```python
from build123d import *

# Parameters (mm, degrees)
F1_DEPTH = 81.5
F2_W     = 1.85
F2_H     = 25.8
F2_H_2   = 4.1
F3_DEPTH = 1.95
F2_W_2   = 7
F4_DEPTH = 8
F5_START = 5
F5_DEPTH = 3


with BuildPart() as f1:
    # F0 (on Top) → F1 (new body)
    with BuildSketch(Plane.XY):
        Polygon((0, -55.5), (0, 0), (10, 0), (10, 9.5), (-5, 9.5), (-5, -50.5), (-80, -50.5), (-80, 9.5), (-95, 9.5), (-95, 0), (-85, 0), (-85, -55.5), align=None)
    extrude(amount=F1_DEPTH)

    # F2 (on face) → F3 (join)
    with BuildSketch(Plane(origin=(0, -50.5, 0), x_dir=(-1, 0, 0), z_dir=(0, 1, 0))):
        Polygon((42.5, 47.4), (42.5, 51.5), (40.65, 51.5), (40.65, 17.5), (42.5, 17.5), (42.5, 21.6), align=None)
        with Locations((43.425, 34.5)):
            Rectangle(F2_W, F2_H)
        with Locations((43.425, 49.45)):
            Rectangle(F2_W, F2_H_2)
        with Locations((43.425, 19.55)):
            Rectangle(F2_W, F2_H_2)
    extrude(amount=F3_DEPTH)

    # F2 (on face) → F4 (join)
    with BuildSketch(Plane(origin=(0, -50.5, 0), x_dir=(-1, 0, 0), z_dir=(0, 1, 0))):
        with Locations((61, 34.5)):
            Rectangle(F2_W_2, F2_H)
        with Locations((24, 34.5)):
            Rectangle(F2_W_2, F2_H)
    extrude(amount=F4_DEPTH)

    # F2 (on face) → F5 (join)
    with BuildSketch(Plane(origin=(0, -50.5, 0), x_dir=(-1, 0, 0), z_dir=(0, 1, 0)).offset(F5_START)):
        Polygon((29.95, 24.05), (29.95, 44.95), (27.5, 47.4), (27.5, 21.6), align=None)
        Polygon((57.5, 21.6), (57.5, 47.4), (55.05, 44.95), (55.05, 24.05), align=None)
    extrude(amount=F5_DEPTH)


solid = f1.part
```
Here's how the part is built. I have some questions about the finished solid (model axes, mm). A direction names the side the tool comes from. Give positions to 0.01 mm unless a question says otherwise; leave off trailing zeros. Order: outer loops, then holes, each group sorted by start corner. A loop starts at its lowest first (then second) coordinate and runs counter-clockwise, first axis right, second up. Notation, with made-up numbers: M 32.25,42 L 68.25,42 A21 ccw 68.25,79 Z; hole C -36,20 d5. An arc over 180 degrees is marked long. Use a Markdown table: item, result. Add a question column.
1. Suppose I cut it at D-D (z = 77). List the corners of the cut face in (x, y) for me, and give its area (4 significant figures).
2. If we mould it in two halves opening along Y, with no side actions, what happens to faces 1 (the flat face through (-64.5, -47, 34)), 2 (the flat face through (-57.5, -48, 34)), 3 (the flat face through (-42, -48.55, 35))? For each: +Y half, -Y half, draft (parallel to the pull), parting line (faces both ways), or undercut.
3. Suppose I cut it at B-B (x = -23). List the corners of the cut face in (y, z) for me.
4. For pin 1 Ø4 at (y, z) = (-45, 33.5) entering from +X; pin 2 Ø1 at (y, z) = (-33, 22) entering from -X; pin 3 Ø4 at (x, z) = (-41.5, 42) entering from +Y; pin 4 Ø6 at (x, y) = (-52.5, -38) entering from +Z, each with a flat end and sliding along its axis, tell me the tip position at first contact or that it passes through.
5. I need wall thicknesses on probe 1 along X at (y, z) = (-21, 28.5); probe 2 along X at (y, z) = (1.5, 41.5); probe 3 along Y at (x, z) = (2.5, 77.5). Which ranges of each line are inside material? Lowest first, please. Write a range as from..to.
6. Suppose I cut it at A-A (y = -9). List the corners of the cut face in (x, z) for me, and give its area (3 significant figures).
7. Suppose I cut it at C-C (z = 39). List the corners of the cut face in (x, y) for me.
8. On a 3-axis mill with a long thin cutter (end or side, diameter ignored), from which of +Z, -Z, +X, -X, +Y, -Y can I reach the whole of each face in a straight line? I mean faces 4 (the flat face through (-60, -42.5, 35)), 5 (the flat face through (5, 0, 40)), 6 (the flat face through (-56, -45.5, 35)), 7 (the flat face through (-90, 0, 40)). Say none if no direction works.
Results list:
| question | item | result |
|---|---|---|
| 1 | outline | M -95,0 L -85,0 L -85,-55.5 L 0,-55.5 L 0,0 L 10,0 L 10,9.5 L -5,9.5 L -5,-50.5 L -80,-50.5 L -80,9.5 L -95,9.5 Z |
| 1 | area | 1,215 mm² |
| 2 | face 1 | draft |
| 2 | face 2 | undercut |
| 2 | face 3 | +Y half |
| 3 | outline | M -55.5,0 L -50.5,0 L -50.5,21.6 L -42.5,21.6 L -42.5,47.4 L -50.5,47.4 L -50.5,81.5 L -55.5,81.5 Z |
| 4 | pin 1 | stops at x = 0 |
| 4 | pin 2 | stops at x = -85 |
| 4 | pin 3 | stops at y = -48.55 |
| 4 | pin 4 | passes through |
| 5 | probe 1 | x = -85..-80, -5..0 |
| 5 | probe 2 | x = -95..-80, -5..10 |
| 5 | probe 3 | y = 0..9.5 |
| 6 | outline | M -85,0 L -80,0 L -80,81.5 L -85,81.5 Z; M -5,0 L 0,0 L 0,81.5 L -5,81.5 Z |
| 6 | area | 815 mm² |
| 7 | outline | M -95,0 L -85,0 L -85,-55.5 L 0,-55.5 L 0,0 L 10,0 L 10,9.5 L -5,9.5 L -5,-50.5 L -20.5,-50.5 L -20.5,-42.5 L -29.95,-42.5 L -29.95,-45.5 L -27.5,-45.5 L -27.5,-50.5 L -40.65,-50.5 L -40.65,-48.55 L -44.35,-48.55 L -44.35,-50.5 L -57.5,-50.5 L -57.5,-45.5 L -55.05,-45.5 L -55.05,-42.5 L -64.5,-42.5 L -64.5,-50.5 L -80,-50.5 L -80,9.5 L -95,9.5 Z |
| 8 | face 4 | +Z, -Z, +Y |
| 8 | face 5 | +Z, -Z, +X, -Y |
| 8 | face 6 | +Z, -Z |
| 8 | face 7 | +Z, -Z, -X, -Y |
